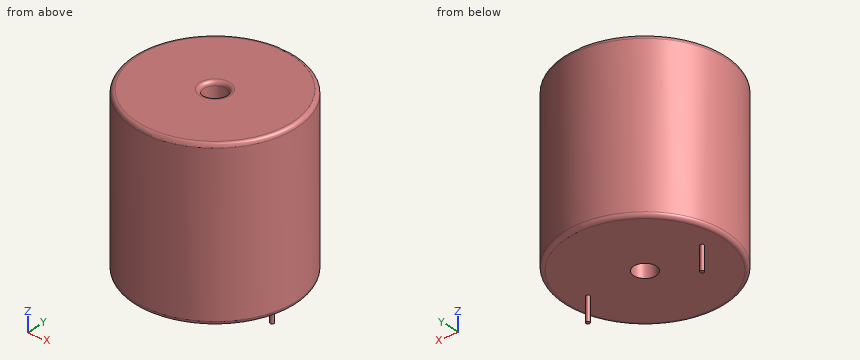
from build123d import *

# Parameters (mm, degrees)
SKETCH001_R       = 0.25
PAD001_DEPTH      = 10.67
PAD001_DEPTH_BACK = 3.5
SKETCH_R          = 10.5
SKETCH_R_2        = 1.46
PAD_DEPTH         = 21.34
FILLET_R          = 0.5


with BuildPart() as pad001:
    # Sketch001 → Pad001 (new body, two sides)
    with BuildSketch(Plane.XY.offset(0.5)) as pad001_sk:
        Circle(SKETCH001_R)
        with Locations((15, 0)):
            Circle(SKETCH001_R)
    extrude(amount=PAD001_DEPTH)
    extrude(pad001_sk.sketch, amount=-PAD001_DEPTH_BACK)


with BuildPart() as obj1:
    # Sketch → Pad (new body)
    with BuildSketch(Plane.XY.offset(0.1)):
        with Locations((7.5, 0)):
            Circle(SKETCH_R)
        with Locations((7.5, 0)):
            Circle(SKETCH_R_2, mode=Mode.SUBTRACT)
    extrude(amount=PAD_DEPTH)

    # Fillet
    fillet_edges = [obj1.edges().sort_by_distance(p)[0] for p in [
        (6.04, 0, 21.44),
        (-3, 0, 21.44),
        (-3, 0, 0.1),
    ]]
    fillet(fillet_edges, radius=FILLET_R)

    # obj1: union Pad001
    add(pad001.part)


solid = obj1.part
Could you check a few things on this model? Use its own coordinates, in mm. Give positions to 0.01 mm unless a question says otherwise; leave off trailing zeros. Order: outer loops, then holes, each group sorted by start corner. A loop starts at its lowest first (then second) coordinate and runs counter-clockwise, first axis right, second up.
Item 1: If we section it at B-B, the plane z = 15.25: Write out the boundary of the cut face in (x, y), plus the area to 3 significant figures.
Item 2: I need wall thicknesses on line 1 (Z direction, x = 5, y = 4); line 2 (Y direction, x = 7.5, z = 13.5); line 3 (X direction, y = 7.75, z = 8). Which ranges of each line are inside material? Lowest first, please.
Item 3: If we section it at A-A, the plane x = 7.5: Write out the boundary of the cut face in (y, z).
Item 4: I'm going to push flat-ended pins straight in: pin 1 (1 mm diameter, centred on x = 13.5, y = 2, fed in from -Z); pin 2 (2 mm diameter, centred on x = 15, z = 12.5, fed in from +Y); pin 3 (2 mm diameter, centred on y = -8.5, z = 5.5, fed in from -X); pin 4 (1.8 mm diameter, centred on x = 7.5, y = 0, fed in from +Z). Where does each tip first touch, or does it pass through?
Values:
1. outline: circle Ø21 at (7.5, 0); hole circle Ø2.92 at (7.5, 0)
1. area: 340 mm2
2. line 1: z = 0.1 to 21.44
2. line 2: y = -10.5 to -1.46, 1.46 to 10.5
2. line 3: x = 0.42 to 14.58
3. outline: (-10.5, 0.6) arc R0.5 ccw to (-10, 0.1) - (-1.46, 0.1) - (-1.46, 20.94) arc R0.5 ccw to (-1.96, 21.44) - (-10, 21.44) arc R0.5 ccw to (-10.5, 20.94) - close; (1.46, 0.1) - (10, 0.1) arc R0.5 ccw to (10.5, 0.6) - (10.5, 20.94) arc R0.5 ccw to (10, 21.44) - (1.96, 21.44) arc R0.5 ccw to (1.46, 20.94) - close
4. pin 1: stops at z = 0.1
4. pin 2: stops at y = 8.25
4. pin 3: stops at x = 0.15
4. pin 4: passes through
